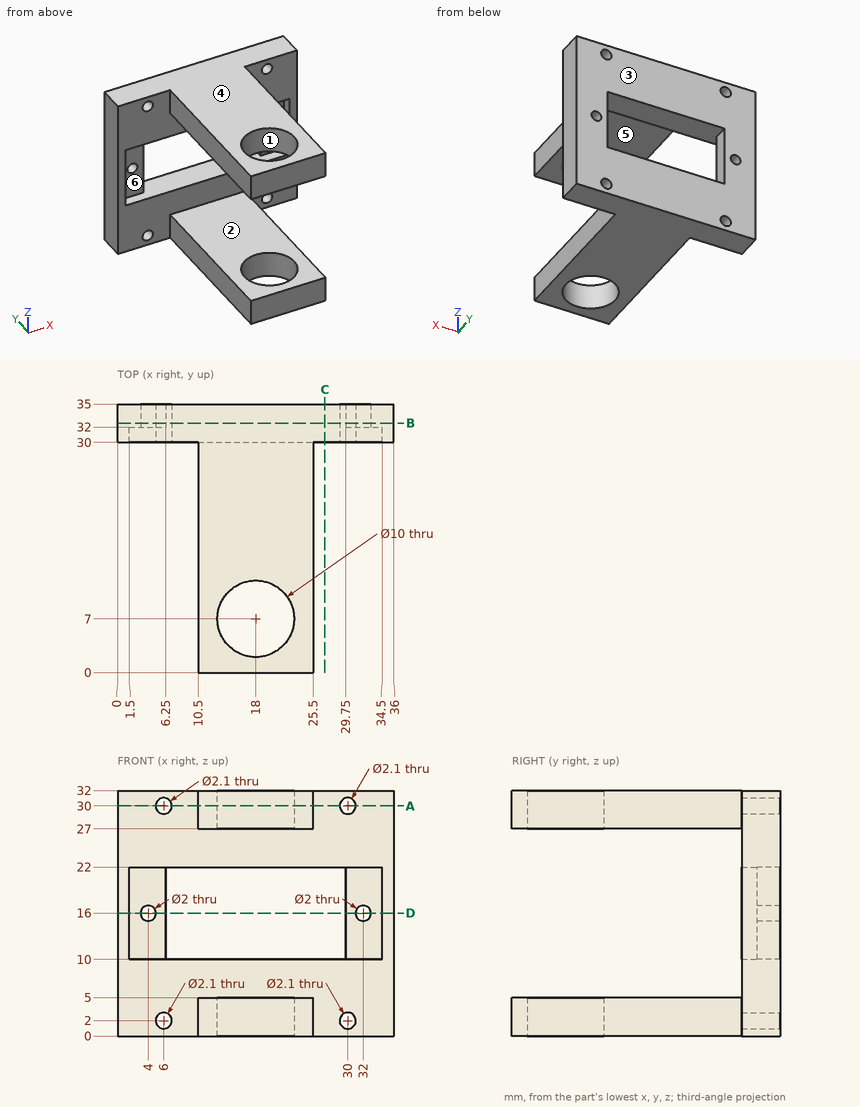
Here's the drawing with two shaded views (mm, measured from the low corner). I have some questions. A direction names the side the tool comes from. Give positions to 0.01 mm unless a question says otherwise; leave off trailing zeros. Order: outer loops, then holes, each group sorted by start corner. A loop starts at its lowest first (then second) coordinate and runs counter-clockwise, first axis right, second up. Notation, with made-up numbers: (35, -32.75) - (39, -32.75) arc R10 ccw to (39, -27.75) - close; hole circle Ø9 at (14, -26.75). An arc over 180 degrees is marked (long way). Use a Markdown table: item, result. Add a question column.
Q1. If we section it at A-A on z = 30: Write out the boundary of the cut face in (x, y), plus the area to 3 significant figures.
Q2. I'm going to push flat-ended pins straight in: pin 1 (2.5 mm diameter, centred on x = 32, z = 16, fed in from -Y); pin 2 (4 mm diameter, centred on y = 19, z = 30.5, fed in from +X); pin 3 (1.5 mm diameter, centred on y = 10.5, z = 1.5, fed in from -X); pin 4 (1.2 mm diameter, centred on x = 32, z = 16, fed in from -Y). Where does each tip first touch, or does it pass through?
Q3. On a 3-axis mill with a long thin cutter (end or side, diameter ignored), from which of +Z, -Z, +X, -X, +Y, -Y can I reach the whole of each face in a straight line? I mean the marked faces 4, 5 and 6. Say none if no direction works.
Q4. If we section it at B-B on y = 32.5: Write out the boundary of the cut face in (x, z), plus the area to 3 significant figures.
Q5. If we section it at D-D on z = 16: Write out the boundary of the cut face in (x, y).
Q6. Please list where these lines run through material, in increasing order: line 1 along X through (y, z) = (31, 30); line 2 along X through (y, z) = (34.2, 16); line 3 along Z through (x, y) = (32, 33).
Q7. If we section it at C-C on x = 27: Write out the boundary of the cut face in (y, z).
Q8. If we mould it in two halves opening along Y, with no side actions, what happens to the marked faces 1, 2 and 3? For each: released by +Y, released by -Y, zero draft, split by the parting line, or undercut.
Answers follow:
| question | item | result |
|---|---|---|
| 1 | outline | (0, 30) - (4.95, 30) - (4.95, 35) - (0, 35) - close; (7.05, 30) - (10.5, 30) - (10.5, 0) - (25.5, 0) - (25.5, 30) - (28.95, 30) - (28.95, 35) - (7.05, 35) - close; (31.05, 30) - (36, 30) - (36, 35) - (31.05, 35) - close; hole circle Ø10 at (18, 7) |
| 1 | area | 530 mm^2 |
| 2 | pin 1 | stops at y = 32 |
| 2 | pin 2 | stops at x = 25.5 |
| 2 | pin 3 | stops at x = 10.5 |
| 2 | pin 4 | passes through |
| 3 | face 4 | +Z, +X, -X, +Y, -Y |
| 3 | face 5 | +X, -X, -Y |
| 3 | face 6 | -Y |
| 4 | outline | (0, 0) - (36, 0) - (36, 32) - (0, 32) - close; hole circle Ø2 at (4, 16); hole circle Ø2.1 at (6, 2); hole circle Ø2.1 at (6, 30); hole (6.25, 10) - (29.75, 10) - (29.75, 22) - (6.25, 22) - close; hole circle Ø2.1 at (30, 2); hole circle Ø2.1 at (30, 30); hole circle Ø2 at (32, 16) |
| 4 | area | 850 mm^2 |
| 5 | outline | (0, 30) - (1.5, 30) - (1.5, 32) - (3, 32) - (3, 35) - (0, 35) - close; (5, 32) - (6.25, 32) - (6.25, 35) - (5, 35) - close; (29.75, 32) - (31, 32) - (31, 35) - (29.75, 35) - close; (33, 32) - (34.5, 32) - (34.5, 30) - (36, 30) - (36, 35) - (33, 35) - close |
| 6 | line 1 | x = 0 to 4.95, 7.05 to 28.95, 31.05 to 36 |
| 6 | line 2 | x = 0 to 3, 5 to 6.25, 29.75 to 31, 33 to 36 |
| 6 | line 3 | z = 0 to 15, 17 to 32 |
| 7 | outline | (30, 0) - (35, 0) - (35, 10) - (30, 10) - close; (30, 22) - (35, 22) - (35, 32) - (30, 32) - close |
| 8 | face 1 | undercut |
| 8 | face 2 | zero draft |
| 8 | face 3 | released by +Y |
